```python
from build123d import *

# Parameters (mm, degrees)
SKETCH1_R                  = 11.1125
EXTRUDE1_DEPTH             = 12.7
BUSHING_SIDE_FILLETS_R     = 0.79375
MOUNT_SIDE_FILLETS_R       = 0.79375
F_1_4_MOUNTING_HOLES_D     = 5.1054
F_1_4_MOUNTING_HOLES_DEPTH = 19.05
F_1_4_MOUNTING_HOLES_TIP   = 1.533816902
EXTRUDE2_DEPTH             = 51.649420448


with BuildPart() as part:
    # Sketch1 → Extrude1 (new, symmetric)
    with BuildSketch(Plane(origin=(0, 0, 0), x_dir=(1, 0, 0), z_dir=(0, 0, -1))):
        with BuildLine():
            Line((-17.705953405, 40.0837), (17.705953405, 40.0837))
            Line((17.705953405, 40.0837), (17.705953405, 30.5587))
            Line((17.705953405, 30.5587), (1.5875, 30.5587))
            Line((1.5875, 30.5587), (1.5875, 12.600390619))
            ThreePointArc((1.5875, 12.600390619), (0, -12.7), (-1.5875, 12.600390619))
            Line((-1.5875, 12.600390619), (-1.5875, 30.5587))
            Line((-1.5875, 30.5587), (-17.705953405, 30.5587))
            Line((-17.705953405, 30.5587), (-17.705953405, 40.0837))
        make_face()
        with Locations(Location((0, 0, 0), (0, 0, 180))):
            Circle(SKETCH1_R, mode=Mode.SUBTRACT)
    extrude(amount=EXTRUDE1_DEPTH, both=True)

    # Bushing-side fillets
    bushing_side_fillets_edges = [part.edges().sort_by_distance(p)[0] for p in [
        (1.5875, -12.600390619, 0),
        (-1.5875, -12.600390619, 0),
    ]]
    fillet(bushing_side_fillets_edges, radius=BUSHING_SIDE_FILLETS_R)

    # Mount-side fillets
    mount_side_fillets_edges = [part.edges().sort_by_distance(p)[0] for p in [
        (1.5875, -30.5587, 0),
        (-1.5875, -30.5587, 0),
    ]]
    fillet(mount_side_fillets_edges, radius=MOUNT_SIDE_FILLETS_R)

    # 1/4 Mounting holes
    with Locations(Plane.XZ.offset(40.0837)):
        with Locations((-12.7, 0), (12.7, 0)):
            Hole(F_1_4_MOUNTING_HOLES_D / 2, depth=F_1_4_MOUNTING_HOLES_DEPTH)
            with Locations((0, 0, -(F_1_4_MOUNTING_HOLES_DEPTH + F_1_4_MOUNTING_HOLES_TIP / 2))):  # 118° drill point
                Cone(0, F_1_4_MOUNTING_HOLES_D / 2, F_1_4_MOUNTING_HOLES_TIP, mode=Mode.SUBTRACT)

    # Sketch4 → Extrude2 (cut, through all)
    with BuildSketch(Plane(origin=(0, 0, -12.7), x_dir=(-1, 0, 0), z_dir=(0, 0, -1))):
        with BuildLine():
            Line((1.5875, -29.76495), (1.5875, -33.7337))
            ThreePointArc((1.5875, -33.7337), (4.7625, -36.9087), (7.9375, -33.7337))
            Line((7.9375, -33.7337), (7.9375, -30.5587))
            Line((7.9375, -30.5587), (2.38125, -30.5587))
            ThreePointArc((2.38125, -30.5587), (1.819983992, -30.326216008), (1.5875, -29.76495))
        make_face()
        with BuildLine():
            Line((-7.9375, -30.5587), (-2.38125, -30.5587))
            ThreePointArc((-2.38125, -30.5587), (-1.819983992, -30.326216008), (-1.5875, -29.76495))
            Line((-1.5875, -29.76495), (-1.5875, -33.7337))
            ThreePointArc((-1.5875, -33.7337), (-4.7625, -36.9087), (-7.9375, -33.7337))
            Line((-7.9375, -33.7337), (-7.9375, -30.5587))
        make_face()
    extrude(amount=-EXTRUDE2_DEPTH, mode=Mode.SUBTRACT)


solid = part.part
```
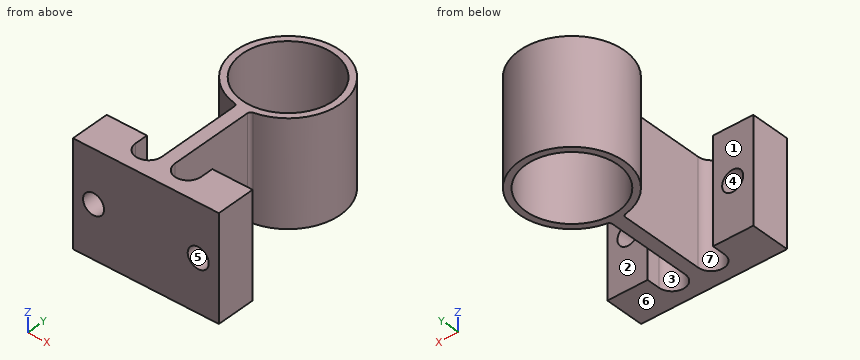
Read the model definition and answer for the solid it produces. Units are mm, in the model's axes. Face numbers are marked on the shaded views. A direction names the side the tool comes from. Coordinates: 2 decimals unless noted, no trailing zeros. Write each loop counter-clockwise with the first axis right and the second up, starting at its lowest first coordinate (ties: lowest second). Pieces come first, ordered by that corner, then holes. Notation, with made-up numbers: (28, -13.5) -> (60, -13.5) arc R18 ccw to (60, 17.5) -> close; hole circle Ø7 at (70, -27.5). An arc over 180 degrees is marked (long way). Write item = value, one per line.
(1) Straight lines are drawn through the part: L1, parallel to X at y = -31, z = -5; L2, parallel to Z at x = 12.7, y = -32.5; L3, parallel to Y at x = -9, z = 2.75. For each, find the intervals that lie inside material, in ascending order. Write a range as from..to.
From the geometry:
L1 = -17.71..-7.94, -1.59..1.59, 7.94..17.71
L2 = -12.7..-2.55, 2.55..12.7
L3 = -40.08..-30.56, -8.96..-6.52, 6.52..8.96
(2) Which of the six approach directions +Z, -Z, +X, -X, +Y, -Y give full straight-line access (tool end or side, diameter ignored) to the marked faces 1, 2 and 3?
From the geometry:
face_1 = +Z, -Z, -X
face_2 = +Z, -Z, +X
face_3 = +Z, -Z
(3) Section B-B on y = 0 is taken. Write down the section's boundary in (x, z), plus the area to 3 significant figures.
From the geometry:
outline = (-12.7, -12.7) -> (-11.11, -12.7) -> (-11.11, 12.7) -> (-12.7, 12.7) -> close; (11.11, -12.7) -> (12.7, -12.7) -> (12.7, 12.7) -> (11.11, 12.7) -> close
area = 80.6 mm2
(4) Section C-C on x = 0 is taken. Write down the section's boundary in (y, z), plus the area to 3 significant figures.
From the geometry:
outline = (-40.08, -12.7) -> (-11.11, -12.7) -> (-11.11, 12.7) -> (-40.08, 12.7) -> close; (11.11, -12.7) -> (12.7, -12.7) -> (12.7, 12.7) -> (11.11, 12.7) -> close
area = 776 mm2
(5) Section A-A on z = 0 is taken. Count the separate pieces of the cut face and the enclosed holes in it, plus the area to 3 significant figures.
From the geometry:
separate_pieces = 3
enclosed_holes = 1
area = 344 mm2
(6) Given pin 1 Ø1 at (y, z) = (-19.5, 4) entering from -X; pin 2 Ø6 at (y, z) = (-20.5, 3) entering from +X; pin 3 Ø4 at (x, z) = (12.7, 0) entering from -Y, each flat-ended and moving along its own axis, determine where each tip first touches the part or whether it passes through.
From the geometry:
pin_1 = -1.59
pin_2 = 1.59
pin_3 = -6.84
(7) For a pull along Z with two mould halves and no side action, classify the marked faces 4, 5, 6 and 7 as +Z half, -Z half, draft (parallel to the pull), parting line (faces both ways), or undercut.
From the geometry:
face_4 = undercut
face_5 = undercut
face_6 = -Z half
face_7 = draft
